from build123d import *

# Parameters (mm, degrees)
F0_R     = 1.2
F1_DEPTH = 10
F2_R     = 1
F3_R     = 11
F4_W     = 12
F4_H     = 7
F5_DEPTH = 10
F6_R     = 0.5


with BuildPart() as f1:
    # F0 (on Top) → F1 (new body)
    with BuildSketch(Plane.XY):
        with BuildLine():
            ThreePointArc((1.9364916731, -3.5), (-2.8284271247, -2.8284271247), (-3.5, 1.9364916731))
            ThreePointArc((-3.5, 1.9364916731), (-1.1055673404, 3.8441801279), (1.9364916731, 3.5))
            Line((1.9364916731, 3.5), (18.9797490537, 3.5))
            Line((18.9797490537, 3.5), (18.9797490537, 5.5))
            Line((18.9797490537, 5.5), (16.9797490537, 5.5))
            Line((16.9797490537, 5.5), (16.9797490537, 4.9))
            Line((16.9797490537, 4.9), (12.9797490537, 4.9))
            Line((12.9797490537, 4.9), (12.9797490537, 5.5))
            Line((12.9797490537, 5.5), (-13.0202509463, 5.5))
            Line((-13.0202509463, 5.5), (-13.0202509463, -4.5))
            Line((-13.0202509463, -4.5), (-13.0202509463, -14.5))
            Line((-13.0202509463, -14.5), (12.9797490537, -14.5))
            Line((12.9797490537, -14.5), (12.9797490537, -5.5))
            Line((12.9797490537, -5.5), (12.9797490537, -4.9))
            Line((12.9797490537, -4.9), (16.9797490537, -4.9))
            Line((16.9797490537, -4.9), (16.9797490537, -5.5))
            Line((16.9797490537, -5.5), (18.9797490537, -5.5))
            Line((18.9797490537, -5.5), (18.9797490537, -3.5))
            Line((18.9797490537, -3.5), (12.9797490537, -3.5))
            Line((12.9797490537, -3.5), (1.9364916731, -3.5))
        make_face()
        with Locations((-9.5, -9.5)):
            Circle(F0_R, mode=Mode.SUBTRACT)
        with Locations((9.5, -9.5)):
            Circle(F0_R, mode=Mode.SUBTRACT)
    extrude(amount=F1_DEPTH)

    # F2
    f2_edges = [f1.edges().sort_by_distance(p)[0] for p in [
        (18.979749, 5.5, 5),
        (18.979749, -5.5, 5),
        (14.979749, 4.9, 10),
        (14.979749, 4.9, 0),
        (12.979749, -4.9, 5),
        (12.979749, -14.5, 5),
        (-13.020251, -14.5, 5),
    ]]
    fillet(f2_edges, radius=F2_R)

    # F3
    f3_edges = [f1.edges().sort_by_distance(p)[0] for p in [
        (-13.020251, 5.5, 5),
    ]]
    fillet(f3_edges, radius=F3_R)

    # F4 (on face) → F5 (cut)
    with BuildSketch(Plane.XY.offset(10)):
        with Locations((0, -9.4900932163)):
            Rectangle(F4_W, F4_H)
    extrude(amount=-F5_DEPTH, mode=Mode.SUBTRACT)

    # F6
    f6_edges = [f1.edges().sort_by_distance(p)[0] for p in [
        (-9.798426, 2.278175, 10),
        (-9.798426, 2.278175, 0),
        (-4, 0, 0),
        (-4, 0, 10),
    ]]
    fillet(f6_edges, radius=F6_R)


solid = f1.part
Check sheet for the modelled part. Datum: model origin and axes. Units: mm. A direction names the side the tool comes from. Round coordinates to 2 decimals unless told otherwise and drop trailing zeros. Loops run counter-clockwise (first coordinate to the right, second up) from the corner with the lowest first, then second, coordinate; pieces in that order, holes last. Notation, with made-up numbers: (80.25, 27.5) -> (89.25, 27.5) arc R13 ccw to (89.25, 51.5) -> close; hole circle Ø5 at (5, 29.5). An arc over 180 degrees is marked (long way). Put each result on its own line as item: value. Start each with the question number.
1. Section check C-C (z = 7.5). Enter the section's corners in (x, y).
2. Section check D-D (x = 14.5). Enter the section's corners in (y, z), plus the area to 3 significant figures.
3. Section check A-A (x = 7). Enter the section's corners in (y, z), plus the area to 3 significant figures.
4. Access from +Z, -Z, +X, -X, +Y, -Y to the whole of each face (thin tool, end or side, straight path). Record for faces 4 (the face through (15, 4.9, 5)), 5 (the face through (12.98, -10, 5)), 6 (the face through (0, -12.99, 5)).
5. Section check B-B (y = -9.5). Enter the section's corners in (x, z).
6. Scan lines: probe 1 along Y at (x, z) = (5.5, 3); probe 2 along Y at (x, z) = (9.5, 4.5); probe 3 along Y at (x, z) = (15, 8). Record each from-to range of solid material in increasing order.
7. Draft check along X on faces 1 (the face through (10, 3.5, 5)), 2 (the face through (18.98, 4, 5)), 3 (the face through (14.952, 4.615, 9.699)). Enter one of: +X half, -X half, draft (parallel to the pull), parting line (faces both ways), or undercut.
8. Gauge pin test, flat ends, axial feed: pin 1 (5.5 mm diameter, centred on y = -10, z = 5.5, fed in from +X); pin 2 (1.8 mm diameter, centred on y = 5, z = 3.5, fed in from -X); pin 3 (1.4 mm diameter, centred on x = 9.5, y = -9.5, fed in from +Z); pin 4 (2.5 mm diameter, centred on x = 15.5, z = 4.5, fed in from -Y). Record the tip position at first contact, or that the pin passes through.
Findings:
1. outline: (-13.02, -13.5) arc R1 ccw to (-12.02, -14.5) -> (11.98, -14.5) arc R1 ccw to (12.98, -13.5) -> (12.98, -5.9) arc R1 cw to (13.98, -4.9) -> (16.98, -4.9) -> (16.98, -5.5) -> (17.98, -5.5) arc R1 ccw to (18.98, -4.5) -> (18.98, -3.5) -> (1.94, -3.5) arc R4 cw (long way) to (1.94, 3.5) -> (18.98, 3.5) -> (18.98, 4.5) arc R1 ccw to (17.98, 5.5) -> (16.98, 5.5) -> (16.98, 4.9) -> (12.98, 4.9) -> (12.98, 5.5) -> (-2.02, 5.5) arc R11 ccw to (-13.02, -5.5) -> close; hole circle Ø2.4 at (-9.5, -9.5); hole (-6, -12.99) -> (6, -12.99) -> (6, -5.99) -> (-6, -5.99) -> close; hole circle Ø2.4 at (9.5, -9.5)
2. outline: (-4.9, 0.5) arc R0.5 ccw to (-4.4, 0) -> (-3.5, 0) -> (-3.5, 10) -> (-4.4, 10) arc R0.5 ccw to (-4.9, 9.5) -> close; (3.5, 0) -> (3.9, 0) arc R1 ccw to (4.9, 1) -> (4.9, 9) arc R1 ccw to (3.9, 10) -> (3.5, 10) -> close
2. area: 27.5 mm^2
3. outline: (-14.5, 0.5) arc R0.5 ccw to (-14, 0) -> (-3.5, 0) -> (-3.5, 10) -> (-14, 10) arc R0.5 ccw to (-14.5, 9.5) -> close; (3.5, 0) -> (5, 0) arc R0.5 ccw to (5.5, 0.5) -> (5.5, 9.5) arc R0.5 ccw to (5, 10) -> (3.5, 10) -> close
3. area: 130 mm^2
4. face 4: +Z, -Z, +Y
4. face 5: +Z, -Z, +X, -Y
4. face 6: +Z, -Z
5. outline: (-13.02, 0.5) arc R0.5 ccw to (-12.52, 0) -> (-10.7, 0) -> (-10.7, 10) -> (-12.52, 10) arc R0.5 ccw to (-13.02, 9.5) -> close; (-8.3, 0) -> (-6, 0) -> (-6, 10) -> (-8.3, 10) -> close; (6, 0) -> (8.3, 0) -> (8.3, 10) -> (6, 10) -> close; (10.7, 0) -> (12.48, 0) arc R0.5 ccw to (12.98, 0.5) -> (12.98, 9.5) arc R0.5 ccw to (12.48, 10) -> (10.7, 10) -> close
6. probe 1: y = -14.5 to -12.99, -5.99 to -3.5, 3.5 to 5.5
6. probe 2: y = -14.5 to -10.7, -8.3 to -3.5, 3.5 to 5.5
6. probe 3: y = -4.9 to -3.5, 3.5 to 4.9
7. face 1: draft
7. face 2: +X half
7. face 3: undercut
8. pin 1: stops at x = 12.98
8. pin 2: stops at x = -7.39
8. pin 3: passes through
8. pin 4: stops at y = -4.9
